Verification items for this drawing (mm, ordinates from the low corner). Round coordinates to 2 decimals unless told otherwise and drop trailing zeros. Order: outer loops, then holes, each group sorted by start corner. A loop starts at its lowest first (then second) coordinate and runs counter-clockwise, first axis right, second up. Notation, with made-up numbers: (-2, 24) - (15, 24) arc R24 cw to (15, 59) - close; hole circle Ø1 at (14.5, 72). An arc over 180 degrees is marked (long way). Return JSON: item names as keys, results as strings. Group by question number.
Q1. Draft check along X on the marked faces 1, 2 and 3. Enter one of: pulls with the +X half, pulls with the -X half, needs draft (parallel to the pull), parting line crosses it, or undercut.
Q2. Sectioned sample at D-D, the plane x = 9. Record the cut outline in (y, z).
Q3. Sectioned sample at A-A, the plane y = 14.95. Record the cut outline in (x, z), then the cut area to 4 significant figures.
Q4. Sectioned sample at B-B, the plane x = 14.95. Record the cut outline in (y, z), then the cut area to 4 significant figures.
Q5. Gauge pin test, flat ends, axial feed: pin 1 Ø12.5 at (x, y) = (14.95, 14.95) entering from +Z; pin 2 Ø1 at (x, z) = (17, 8.5) entering from -Y. Record the tip position at first contact, or that the pin passes through.
Q6. Material ranges on line 1 along Y through (x, z) = (14.95, 7); line 2 along Y through (x, z) = (25.95, 3.25); line 3 along X through (y, z) = (21, 8.5), recorded low to high.
Q7. Sectioned sample at C-C, the plane z = 5.5. Record the cut outline in (x, y).
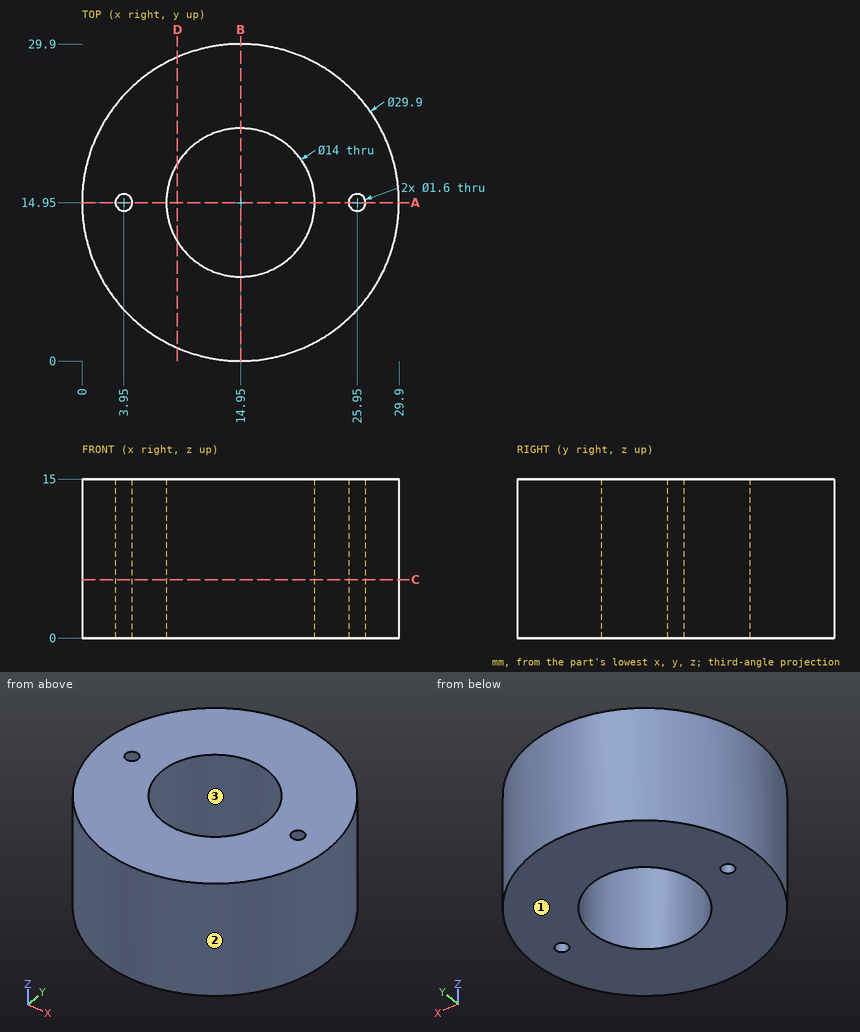
Reply:
{
 "1": {"face 1": "needs draft", "face 2": "parting line crosses it", "face 3": "undercut"},
 "2": {"outline": "(1.24, 0) - (11.26, 0) - (11.26, 15) - (1.24, 15) - close; (18.64, 0) - (28.66, 0) - (28.66, 15) - (18.64, 15) - close"},
 "3": {"outline": "(0, 0) - (3.15, 0) - (3.15, 15) - (0, 15) - close; (4.75, 0) - (7.95, 0) - (7.95, 15) - (4.75, 15) - close; (21.95, 0) - (25.15, 0) - (25.15, 15) - (21.95, 15) - close; (26.75, 0) - (29.9, 0) - (29.9, 15) - (26.75, 15) - close", "area": "190.5 mm^2"},
 "4": {"outline": "(0, 0) - (7.95, 0) - (7.95, 15) - (0, 15) - close; (21.95, 0) - (29.9, 0) - (29.9, 15) - (21.95, 15) - close", "area": "238.5 mm^2"},
 "5": {"pin 1": "through", "pin 2": "y = 0.08"},
 "6": {"line 1": "0 to 7.95, 21.95 to 29.9", "line 2": "4.83 to 14.15, 15.75 to 25.07", "line 3": "1.28 to 11.43, 18.47 to 28.62"},
 "7": {"outline": "circle Ø29.9 at (14.95, 14.95); hole circle Ø1.6 at (3.95, 14.95); hole circle Ø14 at (14.95, 14.95); hole circle Ø1.6 at (25.95, 14.95)"}
}
